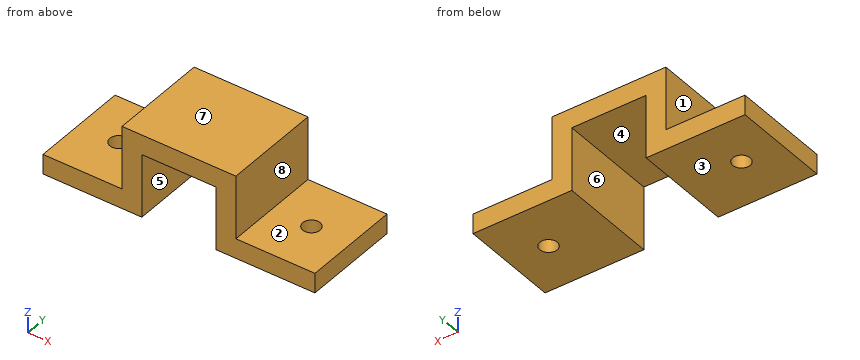
```python
from build123d import *

# Parameters (mm, degrees)
F1_DEPTH = 15.875
F2_R     = 1.397
F3_DEPTH = 25.4


with BuildPart() as f1:
    # F0 (on Front) → F1 (new body)
    with BuildSketch(Plane.XZ):
        Polygon((0.703792, -5.557425), (0.703792, 1.427575), (12.641792, 1.427575), (12.641792, -5.557425), (12.641792, -8.732425), (28.516792, -8.732425), (28.516792, -5.557425), (15.816792, -5.557425), (15.816792, 4.602575), (-2.471208, 4.602575), (-2.471208, 0), (-2.471208, -5.557425), (-15.171208, -5.557425), (-15.171208, -8.732425), (-2.471208, -8.732425), (0.703792, -8.732425), align=None)
    extrude(amount=F1_DEPTH)

    # F2 (on face) → F3 (cut)
    with BuildSketch(Plane.XY.offset(-5.557425)):
        with Locations((-8.821208, -7.9375)):
            Circle(F2_R)
        with Locations((22.166792, -7.9375)):
            Circle(F2_R)
    extrude(amount=-F3_DEPTH, mode=Mode.SUBTRACT)


solid = f1.part
```
For this review, take the finished solid that the model builds, in its own axes (mm). Face numbers are marked on the shaded views. A direction names the side the tool comes from. Round coordinates to 2 decimals unless told otherwise and drop trailing zeros. Write each loop counter-clockwise with the first axis right and the second up, starting at its lowest first coordinate (ties: lowest second). Pieces come first, ordered by that corner, then holes. Notation, with made-up numbers: (44, 71) - (58, 71) arc R19 cw to (58, 84) - close; hole circle Ø4 at (59, 55). An arc over 180 degrees is marked (long way). Put each result on its own line as item: value.
Q1. We need section C-C (x = 22.5). Give the boundary of the cut face in (y, z) (3 decimals).
Solved:
outline: (-15.875, -8.732) - (-9.294, -8.732) - (-9.294, -5.557) - (-15.875, -5.557) - close; (-6.581, -8.732) - (0, -8.732) - (0, -5.557) - (-6.581, -5.557) - close
Q2. We need section D-D (y = -14.5). Give the boundary of the cut face in (x, z), and give its area (3 significant figures).
Solved:
outline: (-15.17, -8.73) - (0.7, -8.73) - (0.7, 1.43) - (12.64, 1.43) - (12.64, -8.73) - (28.52, -8.73) - (28.52, -5.56) - (15.82, -5.56) - (15.82, 4.6) - (-2.47, 4.6) - (-2.47, -5.56) - (-15.17, -5.56) - close
area: 203 mm2
Q3. Machinability: for the marked faces 1, 2, 3 and 4, which of the approach directions +Z, -Z, +X, -X, +Y, -Y give a long, thin tool a straight path to every point of the face, cutting with its end or side? Answer none if there is none.
Solved:
face 1: +Z, -X, +Y, -Y
face 2: +Z, +X, +Y, -Y
face 3: -Z, +X, -X, +Y, -Y
face 4: -Z, +Y, -Y
Q4. Wall thickness on probe 1 along X at (y, z) = (-4.25, 1.25); probe 2 along Z at (x, y) = (-9, -3.75); probe 3 along Z at (x, y) = (5.5, -5.5): over which ranges is each line inside the solid? List them lowest first.
Solved:
probe 1: x = -2.47 to 0.7, 12.64 to 15.82
probe 2: z = -8.73 to -5.56
probe 3: z = 1.43 to 4.6
Q5. We need section B-B (z = -0.25). Give the boundary of the cut face in (x, y) (3 decimals).
Solved:
outline: (-2.471, -15.875) - (0.704, -15.875) - (0.704, 0) - (-2.471, 0) - close; (12.642, -15.875) - (15.817, -15.875) - (15.817, 0) - (12.642, 0) - close
Q6. We need section A-A (z = -7.75). Give the boundary of the cut face in (x, y) (1 decimal), and give its area (3 significant figures).
Solved:
outline: (-15.2, -15.9) - (0.7, -15.9) - (0.7, 0) - (-15.2, 0) - close; (12.6, -15.9) - (28.5, -15.9) - (28.5, 0) - (12.6, 0) - close; hole circle Ø2.8 at (-8.8, -7.9); hole circle Ø2.8 at (22.2, -7.9)
area: 492 mm2
Q7. Insertion check: pin 1 Ø1 at (x, y) = (17.5, -2) entering from +Z; pin 2 Ø6 at (y, z) = (-3, 1.5) entering from +X; pin 3 Ø2 at (x, y) = (22.17, -7.94) entering from -Z. Each pin has a flat end and moves straight along its axis. Give the tip position at first contact, or say it passes through.
Solved:
pin 1: stops at z = -5.56
pin 2: stops at x = 15.82
pin 3: passes through
Q8. Mouldability with a two-part tool opening along X and no side actions: class the marked faces 5, 6, 7 and 8 as released by +X, released by -X, zero draft, split by the parting line, or undercut.
Solved:
face 5: undercut
face 6: undercut
face 7: zero draft
face 8: released by +X
